For this review, take the finished solid that the model builds, in its own axes (mm). A direction names the side the tool comes from. Round coordinates to 2 decimals unless told otherwise and drop trailing zeros. Write each loop counter-clockwise with the first axis right and the second up, starting at its lowest first coordinate (ties: lowest second). Pieces come first, ordered by that corner, then holes. Notation, with made-up numbers: M 44.5,-10.5 L 52.5,-10.5 A30 cw 52.5,21.5 Z; hole C 22.25,56.5 d1. An arc over 180 degrees is marked long. Write each question's results on one line, items separated by ' | '. Start each with the question number.
```python
from build123d import *

# Parameters (mm, degrees)
SKETCH1_R               = 29
BOSS_EXTRUDE1_DEPTH     = 60
CUT_EXTRUDE1_DEPTH      = 73.677369242
CUT_EXTRUDE1_DEPTH_BACK = 73.677369242
CUT_EXTRUDE3_DEPTH      = 8
CUT_EXTRUDE3_DEPTH_BACK = 8
CUT_EXTRUDE4_REACH      = 74.677
SKETCH7_R               = 3.5


with BuildPart() as part:
    # Sketch1 → Boss-Extrude1 (new body)
    with BuildSketch(Plane(origin=(0, 0, 0), x_dir=(1, 0, 0), z_dir=(0, 1, 0))):
        with Locations(Location((0, 0, 0), (0, 0, 270))):
            Circle(SKETCH1_R)
    extrude(amount=BOSS_EXTRUDE1_DEPTH)

    # Sketch2 → Cut-Extrude1 (cut, two sides: drawn at the far end of the back side and taken through both)
    with BuildSketch(Plane.XY.offset(-CUT_EXTRUDE1_DEPTH_BACK)):
        Polygon((-12, 60), (29, 36.328638963), (29, 60), align=None)
    extrude(amount=CUT_EXTRUDE1_DEPTH + CUT_EXTRUDE1_DEPTH_BACK, mode=Mode.SUBTRACT)

    # Sketch6 → Cut-Extrude3 (cut, two sides: drawn at the far end of the back side and taken through both)
    with BuildSketch(Plane.XY.offset(-CUT_EXTRUDE3_DEPTH_BACK)):
        Polygon((15.143593539, 44.328638963), (29, 36.328638963), (29, 0), (15.143593539, 0), align=None)
    extrude(amount=CUT_EXTRUDE3_DEPTH + CUT_EXTRUDE3_DEPTH_BACK, mode=Mode.SUBTRACT)

    # Sketch7 → Cut-Extrude4 (cut, up to next)
    with BuildSketch(Plane(origin=(0, 60, 0), x_dir=(1, 0, 0), z_dir=(0, 1, 0)), mode=Mode.PRIVATE) as cut_extrude4_sk1:
        with Locations(Location((-21, 0, 0), (0, 0, 270))):
            Circle(SKETCH7_R)
    cut_extrude4_tool1 = extrude(cut_extrude4_sk1.sketch, amount=-CUT_EXTRUDE4_REACH, mode=Mode.PRIVATE) & part.part
    add(cut_extrude4_tool1.solids().sort_by_distance((-21, 60, 0))[0], mode=Mode.SUBTRACT)


solid = part.part
```
Item 1: For faces 1 (the flat face through (22, 22, 8)), 2 (the flat face through (-17, 60, 0)), list the 3-axis set-ups (+Z, -Z, +X, -X, +Y, -Y) from which the entire face can be reached by the end or side of a thin tool; tool diameter is ignored.
Item 2: We need section A-A on y = 31. State the section outline as (x, z) points.
Item 3: Insertion check: P1, Ø8, axis at y = 23, z = 9.5, coming from the -X side; P2, Ø12, axis at x = 16.5, y = 15, coming from the -Z side; P3, Ø1, axis at y = 44.5, z = -11.5, coming from the -X side. Each pin has a flat end and moves straight along its axis. Give the tip position at first contact, or say it passes through.
Item 4: We need section B-B on z = 0. State the section outline as (x, y) points.
Item 5: Mouldability with a two-part tool opening along Z and no side actions: class faces 3 (the cylindrical face through (-17.53, 30.42, -0.46)), 4 (the flat face through (0, 0, 0)), 5 (the cylindrical face through (-28.977, 29.58, -1.162)), 6 (the flat face through (22, 22, -8)) as pulls with the +Z half, pulls with the -Z half, needs draft (parallel to the pull), parting line crosses it, or undercut.
Item 6: We need section D-D on x = 18.5. State the section outline as (y, z) points, then the cut area to 3 significant figures.
Item 7: We need section C-C on x = -21. State the section outline as (y, z) points.
Item 8: For probe 1 along X at (y, z) = (13, 0); probe 2 along Z at (x, y) = (1, 7); probe 3 along Z at (x, y) = (-24, 3), list the stretches that pass through material, from the lowest coordinate up.
Numbers:
1) face 1: +X, +Y, -Y | face 2: +Z, -Z, +X, -X, +Y
2) outline: M 15.14,-8 L 15.14,8 L 27.87,8 A29 ccw long 27.87,-8 Z; hole C -21,0 d7
3) P1: stops at x = -28.47 | P2: stops at z = -27.03 | P3: stops at x = -26.83
4) outline: M -29,0 L -24.5,0 L -24.5,60 L -29,60 Z; M -17.5,0 L 15.14,0 L 15.14,44.33 L -12,60 L -17.5,60 Z
5) face 3: undercut | face 4: needs draft | face 5: parting line crosses it | face 6: undercut
6) outline: M 0,-22.33 L 42.39,-22.33 L 42.39,-8 L 0,-8 Z; M 0,8 L 42.39,8 L 42.39,22.33 L 0,22.33 Z | area: 1,220 mm^2
7) outline: M 0,-20 L 60,-20 L 60,-3.5 L 0,-3.5 Z; M 0,3.5 L 60,3.5 L 60,20 L 0,20 Z
8) probe 1: x = -29 to -24.5, -17.5 to 15.14 | probe 2: z = -28.98 to 28.98 | probe 3: z = -16.28 to -1.8, 1.8 to 16.28
